Model file for the job. Use its own axes, mm. Face numbers are marked on the shaded views. A direction names the side the tool comes from. Give positions to 0.01 mm unless a question says otherwise; leave off trailing zeros. Loops run counter-clockwise (first coordinate to the right, second up) from the corner with the lowest first, then second, coordinate; pieces in that order, holes last. Notation, with made-up numbers: M 53.25,11.5 L 93.25,11.5 A15 cw 93.25,29.5 Z; hole C 71,-8 d4. An arc over 180 degrees is marked long. Answer in a Markdown table with one row per item.
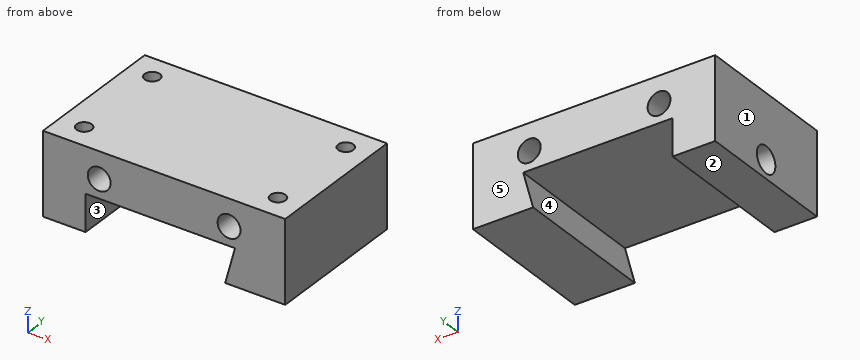
```python
from build123d import *

# Parameters (mm, degrees)
F0_W     = 31.75
F0_H     = 19.05
F1_DEPTH = 10.795
F3_DEPTH = 25.4
F5_D     = 3
F7_D     = 2
F7_DEPTH = 6.35
F7_TIP   = 0.600860619
F9_D     = 3.4544
F9_DEPTH = 6.35
F9_TIP   = 1.0378064612


with BuildPart() as f1:
    # F0 (on Top) → F1 (new body)
    with BuildSketch(Plane.XY):
        with Locations((15.875, 9.525)):
            Rectangle(F0_W, F0_H)
    extrude(amount=F1_DEPTH)

    # F2 (on face) → F3 (cut)
    with BuildSketch(Plane.XZ):
        Polygon((23.876, 0), (25.1691228027, 4.826), (5.588, 4.826), (5.588, 0), align=None)
    extrude(amount=-F3_DEPTH, mode=Mode.SUBTRACT)

    # F5 (through all)
    with Locations(Plane.XZ):
        with Locations((7.366, 7.2898), (24.384, 7.2898)):
            Hole(F5_D / 2)

    # F7
    with Locations(Plane.XY.offset(10.795)):
        with Locations((3.2063322142, 15.875), (3.175, 3.175), (28.575, 15.875), (28.575, 3.175)):
            Hole(F7_D / 2, depth=F7_DEPTH)
            with Locations((0, 0, -(F7_DEPTH + F7_TIP / 2))):  # 118° drill point
                Cone(0, F7_D / 2, F7_TIP, mode=Mode.SUBTRACT)

    # F9
    with Locations(Plane(origin=(0, 0, 0), x_dir=(0, -1, 0), z_dir=(-1, 0, 0))):
        with Locations((-9.525, 2.413)):
            Hole(F9_D / 2, depth=F9_DEPTH)
            with Locations((0, 0, -(F9_DEPTH + F9_TIP / 2))):  # 118° drill point
                Cone(0, F9_D / 2, F9_TIP, mode=Mode.SUBTRACT)


solid = f1.part
```
Q1. Saw through at B-B (y = 10.25). Give the cut face in (x, z) (3 decimals), and give its area (3 significant figures).
Reported:
| item | result |
|---|---|
| outline | M 0,0 L 5.588,0 L 5.588,0.845 L 0,0.845 Z; M 0,3.981 L 5.588,3.981 L 5.588,4.826 L 25.169,4.826 L 23.876,0 L 31.75,0 L 31.75,10.795 L 0,10.795 Z; hole C 7.366,7.29 d3; hole C 24.384,7.29 d3 |
| area | 220 mm² |
Q2. Saw through at C-C (x = 7.5). Give the cut face in (y, z) (3 decimals), and give its area (3 significant figures).
Reported:
| item | result |
|---|---|
| outline | M 0,4.826 L 19.05,4.826 L 19.05,5.796 L 0,5.796 Z; M 0,8.784 L 19.05,8.784 L 19.05,10.795 L 0,10.795 Z |
| area | 56.8 mm² |
Q3. Probe probe 1 along X at (y, z) = (16, 9); probe 2 along X at (y, z) = (16.5, 4.5); probe 3 along Z at (x, y) = (7.5, 10.5) (3 decimals). List the from-to ranges inside material, lowest first.
Reported:
| item | result |
|---|---|
| probe 1 | 0 to 2.21, 4.2 to 27.58, 29.57 to 31.75 |
| probe 2 | 0 to 2.43, 3.99 to 5.59, 25.08 to 27.79, 29.36 to 31.75 |
| probe 3 | 4.826 to 5.796, 8.784 to 10.795 |
Q4. Saw through at D-D (z = 9.75). Give the cut face in (x, y) (3 decimals), and give its area (3 significant figures).
Reported:
| item | result |
|---|---|
| outline | M 0,0 L 31.75,0 L 31.75,19.05 L 0,19.05 Z; hole C 3.175,3.175 d2; hole C 3.206,15.875 d2; hole C 28.575,3.175 d2; hole C 28.575,15.875 d2 |
| area | 592 mm² |
Q5. Saw through at A-A (z = 3.5). Give the cut face in (x, y).
Reported:
| item | result |
|---|---|
| outline | M 0,0 L 5.59,0 L 5.59,8.18 L 0,8.18 Z; M 0,10.87 L 5.59,10.87 L 5.59,19.05 L 0,19.05 Z; M 24.81,0 L 31.75,0 L 31.75,19.05 L 24.81,19.05 Z |
Q6. 3-axis set-ups, long thin cutter, end or side, ignore diameter. For the marked faces 4 and 5: which of +Z, -Z, +X, -X, +Y, -Y reach the whole face in a straight line?
Reported:
| item | result |
|---|---|
| face 4 | +Y, -Y |
| face 5 | +Z, -Z, +X, -X, +Y |
Q7. Drop flat-ended pins along their axis: pin 1 (1 mm diameter, centred on y = 3.5, z = 8, fed in from -X); pin 2 (2 mm diameter, centred on y = 9.525, z = 2.413, fed in from -X). Give the stop position or say it passes through.
Reported:
| item | result |
|---|---|
| pin 1 | x = 0 |
| pin 2 | x = 24.25 |
Q8. Mould opens along X. For the marked faces 1, 2 and 3 say: released by +X, released by -X, zero draft, split by the parting line, or undercut.
Reported:
| item | result |
|---|---|
| face 1 | released by -X |
| face 2 | zero draft |
| face 3 | undercut |
